from build123d import *

# Parameters (mm, degrees)
SKETCH1_W               = 30
SKETCH1_H               = 36
BOSS_EXTRUDE1_DEPTH     = 30
SKETCH3_R               = 12.375
CUT_EXTRUDE1_DEPTH      = 40
SKETCH5_R               = 1.875
CUT_EXTRUDE2_DEPTH      = 40
CUT_EXTRUDE3_START      = 15
SKETCH7_W               = 36
SKETCH7_H               = 15
CUT_EXTRUDE3_DEPTH      = 31
BOSS_EXTRUDE2_DEPTH     = 38
SKETCH9_R               = 0.5
SKETCH9_W               = 22.5
SKETCH9_H               = 12.5
CUT_EXTRUDE4_DEPTH      = 10
SKETCH10_W              = 31.281266854
SKETCH10_H              = 4.861672308
CUT_EXTRUDE6_DEPTH      = 31.375
CUT_EXTRUDE6_DEPTH_BACK = 6.625


with BuildPart() as part:
    # Sketch1 → Boss-Extrude1 (new body)
    with BuildSketch(Plane(origin=(0, 0, 0), x_dir=(1, 0, 0), z_dir=(0, 1, 0))):
        Rectangle(SKETCH1_W, SKETCH1_H)
    extrude(amount=BOSS_EXTRUDE1_DEPTH)

    # Sketch3 → Cut-Extrude1 (cut)
    with BuildSketch(Plane(origin=(15, 0, 0), x_dir=(0, 0, -1), z_dir=(1, 0, 0))):
        with Locations((0, 15)):
            Circle(SKETCH3_R)
    extrude(amount=-CUT_EXTRUDE1_DEPTH, mode=Mode.SUBTRACT)

    # Sketch5 → Cut-Extrude2 (cut)
    with BuildSketch(Plane(origin=(0, 30, 0), x_dir=(1, 0, 0), z_dir=(0, 1, 0))):
        with Locations((-12.25, 15.25)):
            Circle(SKETCH5_R)
        with Locations((-12.25, -15.25)):
            Circle(SKETCH5_R)
        with Locations((12.25, -15.25)):
            Circle(SKETCH5_R)
        with Locations((12.25, 15.25)):
            Circle(SKETCH5_R)
    extrude(amount=-CUT_EXTRUDE2_DEPTH, mode=Mode.SUBTRACT)

    # Sketch7 → Cut-Extrude3 (cut, through all)
    with BuildSketch(Plane(origin=(0, 0, 0), x_dir=(0, 0, -1), z_dir=(1, 0, 0)).offset(CUT_EXTRUDE3_START)):
        with Locations((0, 7.5)):
            Rectangle(SKETCH7_W, SKETCH7_H)
    extrude(amount=-CUT_EXTRUDE3_DEPTH, mode=Mode.SUBTRACT)

    # Sketch8 → Boss-Extrude2 (add)
    with BuildSketch(Plane(origin=(15, 0, 0), x_dir=(0, 0, -1), z_dir=(1, 0, 0))):
        Polygon((-18, 30), (18, 30), (18, 27.331397605), (18, 15), (12.375, 15), (12.375, 27.331397605), (-12.375, 27.331397605), (-12.375, 15), (-18, 15), (-18, 27.331397605), align=None)
    extrude(amount=BOSS_EXTRUDE2_DEPTH)

    # Sketch9 → Cut-Extrude4 (cut)
    with BuildSketch(Plane(origin=(0, 30, 0), x_dir=(1, 0, 0), z_dir=(0, 1, 0))):
        with Locations((20.532846914, 0)):
            Circle(SKETCH9_R)
        with Locations((47.532846914, 0)):
            Circle(SKETCH9_R)
        with Locations((34, 0)):
            Rectangle(SKETCH9_W, SKETCH9_H)
    extrude(amount=-CUT_EXTRUDE4_DEPTH, mode=Mode.SUBTRACT)

    # Sketch10 → Cut-Extrude6 (cut, two sides)
    with BuildSketch(Plane(origin=(0, 0, 12.375), x_dir=(-1, 0, 0), z_dir=(0, 0, -1))) as cut_extrude6_sk:
        with Locations((-37.359366573, 17.430836154)):
            Rectangle(SKETCH10_W, SKETCH10_H)
    extrude(amount=CUT_EXTRUDE6_DEPTH, mode=Mode.SUBTRACT)
    extrude(cut_extrude6_sk.sketch, amount=-CUT_EXTRUDE6_DEPTH_BACK, mode=Mode.SUBTRACT)


solid = part.part
Work out the finished part from the listing and answer in its coordinate system (mm). A direction names the side the tool comes from. Give positions to 0.01 mm unless a question says otherwise; leave off trailing zeros. Write each loop counter-clockwise with the first axis right and the second up, starting at its lowest first coordinate (ties: lowest second). Pieces come first, ordered by that corner, then holes.
Q1. The part is cut by section A-A on x = 27. Give the vertices of the cut face in (y, z) (3 decimals), and give its area (3 significant figures).
Answer:
outline: (19.862, -18) - (30, -18) - (30, -6.25) - (27.331, -6.25) - (27.331, -12.375) - (19.862, -12.375) - close; (19.862, 12.375) - (27.331, 12.375) - (27.331, 6.25) - (30, 6.25) - (30, 18) - (19.862, 18) - close
area: 147 mm2
Q2. Straight lines are drawn through the part: L1, parallel to X at y = 23.75, z = 15.25 (3 decimals); L2, parallel to X at y = 28, z = 0; L3, parallel to Z at x = -12.25, y = 20.75 (3 decimals). For each, find the intervals that lie inside material, in ascending order.
Answer:
L1: x = -15 to -14.125, -10.375 to 10.375, 14.125 to 53
L2: x = -15 to 20.03, 21.03 to 22.75, 45.25 to 47.03, 48.03 to 53
L3: z = -18 to -17.125, -13.375 to -10.958, 10.958 to 13.375, 17.125 to 18
Q3. The part is cut by section D-D on z = 15.25. Give the vertices of the cut face in (x, y) (3 decimals).
Answer:
outline: (-15, 15) - (-14.125, 15) - (-14.125, 30) - (-15, 30) - close; (-10.375, 15) - (10.375, 15) - (10.375, 30) - (-10.375, 30) - close; (14.125, 15) - (21.719, 15) - (21.719, 19.862) - (53, 19.862) - (53, 30) - (14.125, 30) - close
Q4. A tool of negligible diameter and unlimited length cuts with its end or side. For faces 4 (the face through (21.719, 17, -15)), 5 (the face through (34, 29, 6.25)), 6 (the face through (30, 22, -12.375)), from which of +Z, -Z, +X, -X, +Y, -Y can it reach the whole face along a straight path? Write none if from no direction.
Answer:
face 4: +Z, -Z, +X, -Y
face 5: +Y, -Y
face 6: +X, -Y
Q5. For a pull along Z with two mould halves and no side action, classify faces 1 (the face through (19, 24, -18)), 2 (the face through (53, 28, 0)), 3 (the face through (13.26, 22.6, 13.67)) as released by +Z, released by -Z, zero draft, split by the parting line, or undercut.
Answer:
face 1: released by -Z
face 2: zero draft
face 3: undercut
Q6. The part is cut by section C-C on y = 21. Give the vertices of the cut face in (x, z) (3 decimals), and give its area (3 significant figures).
Answer:
outline: (-15, -18) - (53, -18) - (53, -12.375) - (15, -12.375) - (15, -10.823) - (-15, -10.823) - close; (-15, 10.823) - (15, 10.823) - (15, 12.375) - (53, 12.375) - (53, 18) - (-15, 18) - close; hole circle Ø3.75 at (-12.25, -15.25); hole circle Ø3.75 at (-12.25, 15.25); hole circle Ø3.75 at (12.25, -15.25); hole circle Ø3.75 at (12.25, 15.25)
area: 814 mm2
Q7. Given pin 1 (2.5 mm diameter, centred on y = 17, z = -15, fed in from +X); pin 2 (8 mm diameter, centred on x = 44.5, z = 8.5, fed in from -Y); pin 3 (2 mm diameter, centred on x = -12.25, z = 15.25, fed in from +Y), each flat-ended and moving along its own axis, determine where each tip first touches the part or whether it passes through.
Answer:
pin 1: stops at x = 21.72
pin 2: stops at y = 19.86
pin 3: passes through
Q8. The part is cut by section B-B on x = 12.25. Give the vertices of the cut face in (y, z) (3 decimals), and give its area (3 significant figures).
Answer:
outline: (15, -18) - (30, -18) - (30, -17.125) - (15, -17.125) - close; (15, -13.375) - (30, -13.375) - (30, 13.375) - (15, 13.375) - (15, 12.375) arc R12.375 cw to (15, -12.375) - close; (15, 17.125) - (30, 17.125) - (30, 18) - (15, 18) - close
area: 187 mm2
